Input: part model. Units: mm. Frame: model coordinates. A direction names the side the tool comes from. Coordinates: 2 decimals unless noted, no trailing zeros. Write each loop counter-clockwise with the first axis right and the second up, starting at its lowest first coordinate (ties: lowest second). Pieces come first, ordered by that corner, then holes. Notation, with made-up numbers: M 59.5,-6.75 L 86.5,-6.75 A19 ccw 86.5,30.25 Z; hole C -3,27 d2. An arc over 180 degrees is marked long. Use CSV: the item, a comma, the result in double quotes.
```python
from build123d import *

# Parameters (mm, degrees)
SKETCH_1_W      = 112
SKETCH_1_H      = 60
SKETCH_1_R      = 1.5
SKETCH_1_W_2    = 3
SKETCH_1_H_2    = 20
EXTRUDE_1_DEPTH = 6


with BuildPart() as part:
    # 草图1 → 凸台-拉伸1 (new body)
    with BuildSketch(Plane(origin=(0, 0, 0), x_dir=(1, 0, 0), z_dir=(0, 1, 0))):
        with Locations((56, -30)):
            Rectangle(SKETCH_1_W, SKETCH_1_H)
        with Locations(Location((75, -4.5, 0), (0, 0, 270))):
            Circle(SKETCH_1_R, mode=Mode.SUBTRACT)
        with Locations(Location((37, -4.5, 0), (0, 0, 270))):
            Circle(SKETCH_1_R, mode=Mode.SUBTRACT)
        with Locations(Location((75, -55.5, 0), (0, 0, 270))):
            Circle(SKETCH_1_R, mode=Mode.SUBTRACT)
        with Locations(Location((37, -55.5, 0), (0, 0, 270))):
            Circle(SKETCH_1_R, mode=Mode.SUBTRACT)
        with Locations((4.5, -18)):
            Rectangle(SKETCH_1_W_2, SKETCH_1_H_2, mode=Mode.SUBTRACT)
        with Locations((4.5, -42)):
            Rectangle(SKETCH_1_W_2, SKETCH_1_H_2, mode=Mode.SUBTRACT)
        with Locations((107.5, -18)):
            Rectangle(SKETCH_1_W_2, SKETCH_1_H_2, mode=Mode.SUBTRACT)
        with Locations((107.5, -42)):
            Rectangle(SKETCH_1_W_2, SKETCH_1_H_2, mode=Mode.SUBTRACT)
        with Locations((12.5, -42)):
            Rectangle(SKETCH_1_W_2, SKETCH_1_H_2, mode=Mode.SUBTRACT)
        with Locations((12.5, -18)):
            Rectangle(SKETCH_1_W_2, SKETCH_1_H_2, mode=Mode.SUBTRACT)
        with Locations((99.5, -18)):
            Rectangle(SKETCH_1_W_2, SKETCH_1_H_2, mode=Mode.SUBTRACT)
        with Locations((99.5, -42)):
            Rectangle(SKETCH_1_W_2, SKETCH_1_H_2, mode=Mode.SUBTRACT)
    extrude(amount=EXTRUDE_1_DEPTH)


solid = part.part
```
1. Mould query, pull axis Z, two halves, no side actions, for faces 1 (the flat face through (112, 3, 30)), 2 (the flat face through (99, 3, 8)). Classes: pulls with the +Z half, pulls with the -Z half, needs draft (parallel to the pull), parting line crosses it, or undercut.
Resolved:
face 1,"needs draft"
face 2,"undercut"
2. Material intervals for line 1 (X direction, y = 2, z = 55.5); line 2 (Z direction, x = 75, y = 4.2); line 3 (Z direction, x = 100.5, y = 5.15), sorted ascending. Write a range as [from, to].
Resolved:
line 1,"x = [0, 35.5], [38.5, 73.5], [76.5, 112]"
line 2,"z = [0, 3], [6, 54], [57, 60]"
line 3,"z = [0, 8], [28, 32], [52, 60]"
3. Contact query for a flat-ended pin moving along its axis: pin 1 Ø2.5 at (x, z) = (37, 55.5) entering from +Y. Output: stop coordinate, or through.
Resolved:
pin 1,"passes through"
4. Access query for faces 3 (the flat face through (12, 3, 32)), 4 (the flat face through (55, 6, 30)). Directions: +Z, -Z, +X, -X, +Y, -Y. A direction counts if a zero-diameter tool reaches every point of the face in a straight line with its end or side. Return the directions, or none.
Resolved:
face 3,"+Y, -Y"
face 4,"+Z, -Z, +X, -X, +Y"
5. Section B-B (x = 37). Return loops of the section in (y, z), then the cut area to 3 significant figures.
Resolved:
outline,"M 0,0 L 6,0 L 6,3 L 0,3 Z; M 0,6 L 6,6 L 6,54 L 0,54 Z; M 0,57 L 6,57 L 6,60 L 0,60 Z"
area,"324 mm^2"
6. Section A-A (z = 36). Return loops of the section in (x, y).
Resolved:
outline,"M 0,0 L 3,0 L 3,6 L 0,6 Z; M 6,0 L 11,0 L 11,6 L 6,6 Z; M 14,0 L 98,0 L 98,6 L 14,6 Z; M 101,0 L 106,0 L 106,6 L 101,6 Z; M 109,0 L 112,0 L 112,6 L 109,6 Z"
7. Section C-C (z = 55.5). Return loops of the section in (x, y).
Resolved:
outline,"M 0,0 L 35.5,0 L 35.5,6 L 0,6 Z; M 38.5,0 L 73.5,0 L 73.5,6 L 38.5,6 Z; M 76.5,0 L 112,0 L 112,6 L 76.5,6 Z"
8. Section D-D (y = 2.5). State how many separate pieces and enclosed holes the cut face has, then the cut area to 3 significant figures.
Resolved:
separate pieces,"1"
enclosed holes,"12"
area,"6,210 mm^2"
